Print and shaded views of the part. All mm, measured from the part's lowest x, y and z. Round coordinates to 2 decimals unless told otherwise and drop trailing zeros. Write each loop counter-clockwise with the first axis right and the second up, starting at its lowest first coordinate (ties: lowest second). Pieces come first, ordered by that corner, then holes. Notation, with made-up numbers: (73.5, -19) - (102.5, -19) arc R27 ccw to (102.5, 0) - close; hole circle Ø11 at (-30.75, -30.5). An arc over 180 degrees is marked (long way). Put each result on its own line as item: value. Start each with the question number.
Item 1: Drill centre lines: line 1 (Z direction, x = 143, y = 1.1); line 2 (X direction, y = 1.2, z = 135); line 3 (X direction, y = 0.55, z = 5). Where is each one in solid material? Low to high. Write a range as from..to.
Item 2: Cut at A-A (z = 135). Give the cut face in (x, y).
Item 3: Cut at B-B (x = 5). Give the cut face in (y, z), and give its area (3 significant figures).
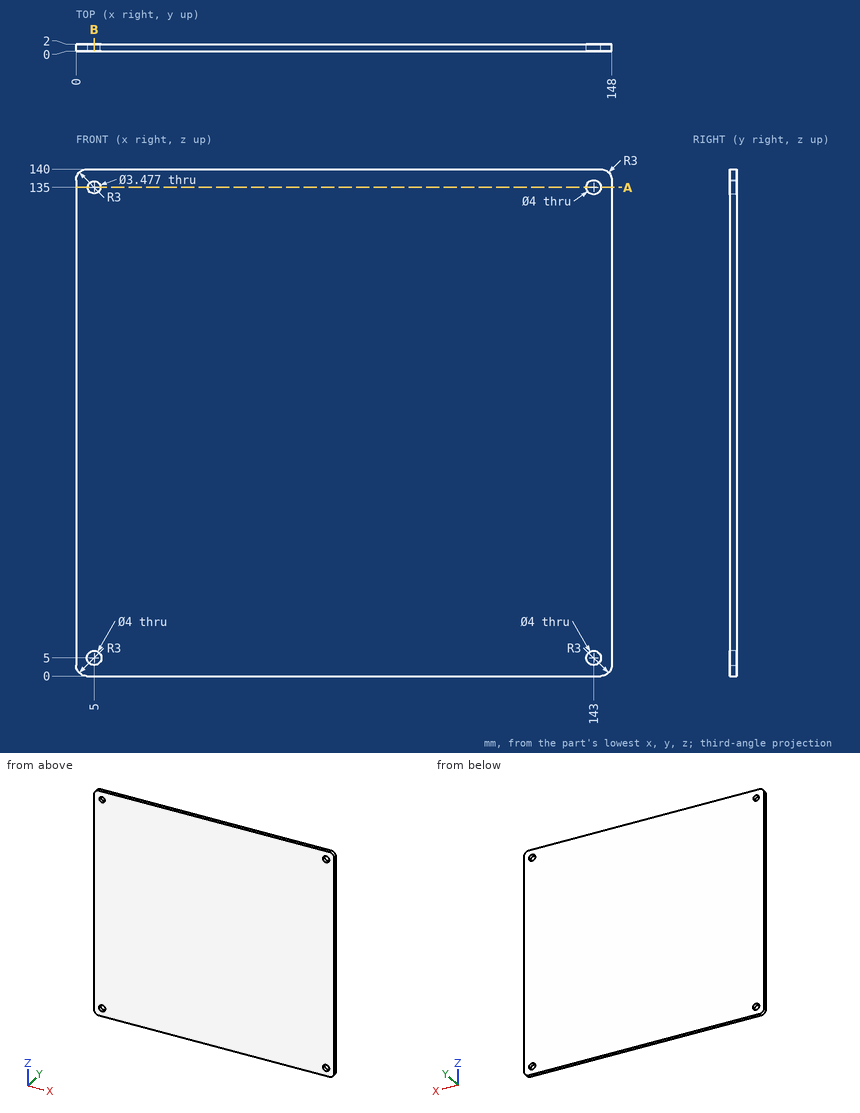
Output values:
1. line 1: 0..3, 7..133, 137..140
1. line 2: 0..3.26, 6.74..141, 145..148
1. line 3: 0..3, 7..141, 145..148
2. outline: (0, 0) - (3.26, 0) - (3.26, 2) - (0, 2) - close; (6.74, 0) - (141, 0) - (141, 2) - (6.74, 2) - close; (145, 0) - (148, 0) - (148, 2) - (145, 2) - close
3. outline: (0, 0) - (2, 0) - (2, 3) - (0, 3) - close; (0, 7) - (2, 7) - (2, 133.26) - (0, 133.26) - close; (0, 136.74) - (2, 136.74) - (2, 140) - (0, 140) - close
3. area: 265 mm2
